Work out the finished part from the listing and answer in its coordinate system (mm). Coordinates: 2 decimals unless noted, no trailing zeros. Loops run counter-clockwise (first coordinate to the right, second up) from the corner with the lowest first, then second, coordinate; pieces in that order, holes last. Notation, with made-up numbers: (21, 9.5) -> (73, 9.5) arc R10 ccw to (73, 14.5) -> close; hole circle Ø6 at (84, 73). An arc over 180 degrees is marked (long way). One line per question, with ' | ' between items.
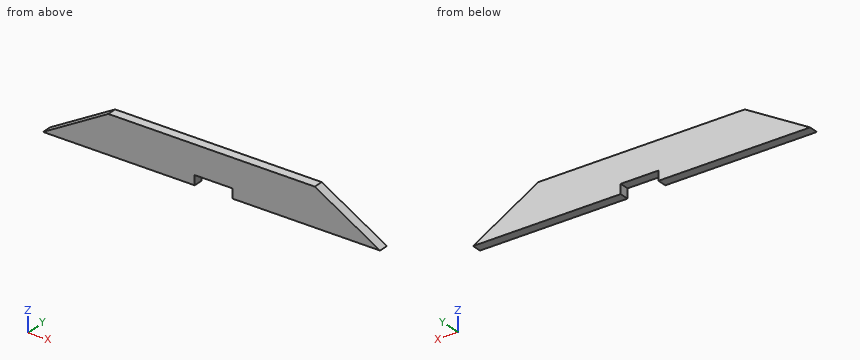
```python
from build123d import *

# Parameters (mm, degrees)
F2_DEPTH = 12.7
F3_W     = 101.6
F3_H     = 25.4
F4_DEPTH = 50


with BuildPart() as f2:
    # F1 (on Front) → F2 (new body, symmetric)
    with BuildSketch(Plane.XZ):
        Polygon((-283.658414, 440.6), (-459.634776, 339), (448.271281, 339), (272.294919, 440.6), align=None)
    extrude(amount=F2_DEPTH, both=True)

    # F3 (on Front) → F4 (cut, symmetric)
    with BuildSketch(Plane.XZ):
        with Locations((-0.2, 351.7)):
            Rectangle(F3_W, F3_H)
    extrude(amount=F4_DEPTH, both=True, mode=Mode.SUBTRACT)


solid = f2.part
```
1) Flat-ended cylindrical pins translate along their axes: pin 1 (10 mm diameter, centred on y = -7, z = 410, fed in from +X); pin 2 (2 mm diameter, centred on y = -5, z = 370.5, fed in from -X). Find the tip coordinate at first contact, or state that the pin passes through.
Check values:
pin 1: stops at x = 333.96 | pin 2: stops at x = -406.81
2) Find section A-A (z = 349.5). Write down the section's boundary in (x, y).
Check values:
outline: (-441.45, -12.7) -> (-51, -12.7) -> (-51, 12.7) -> (-441.45, 12.7) -> close; (50.6, -12.7) -> (430.08, -12.7) -> (430.08, 12.7) -> (50.6, 12.7) -> close
3) Find section D-D (x = -299). Write down the section's boundary in (y, z).
Check values:
outline: (-12.7, 339) -> (12.7, 339) -> (12.7, 431.74) -> (-12.7, 431.74) -> close
4) Find the intervals of material crossed by line 1 along X through (y, z) = (9.25, 358); line 2 along X through (y, z) = (0.75, 344.5) (1 decimal); line 3 along X through (y, z) = (-10, 424.5), in increasing order.
Check values:
line 1: x = -426.73 to -51, 50.6 to 415.36 | line 2: x = -450.1 to -51, 50.6 to 438.7 | line 3: x = -311.54 to 300.18
5) Find section C-C (z = 427). Write down the section's boundary in (x, y).
Check values:
outline: (-307.21, -12.7) -> (295.85, -12.7) -> (295.85, 12.7) -> (-307.21, 12.7) -> close
6) Find section B-B (y = -1.75). Write down the section's boundary in (x, z), plus the area to 3 significant figures.
Check values:
outline: (-459.63, 339) -> (-51, 339) -> (-51, 364.4) -> (50.6, 364.4) -> (50.6, 339) -> (448.27, 339) -> (272.29, 440.6) -> (-283.66, 440.6) -> close | area: 71,800 mm^2
